Part model, mm, in its own coordinate system. A direction names the side the tool comes from. Give positions to 0.01 mm unless a question says otherwise; leave off trailing zeros. Order: outer loops, then holes, each group sorted by start corner. A loop starts at its lowest first (then second) coordinate and runs counter-clockwise, first axis right, second up. Notation, with made-up numbers: M 22.25,-4.75 L 26.25,-4.75 A33 ccw 26.25,32.25 Z; hole C -9,84.25 d3. An arc over 180 degrees is marked long. Return JSON: item names as keys, results as strings.
from build123d import *

# Parameters (mm, degrees)
SKETCH_1_R      = 2.5
SKETCH_1_R_2    = 1.45
EXTRUDE_2_DEPTH = 3


with BuildPart() as part:
    # 草圖1 → 填料-伸長2 (new body)
    with BuildSketch(Plane.XY):
        with BuildLine():
            ThreePointArc((-56.198698673, 17.411107553), (-54.880679188, 14.229127038), (-51.698698673, 12.911107553))
            Line((-51.698698673, 12.911107553), (-48.698698673, 12.911107553))
            Line((-48.698698673, 12.911107553), (-48.698698673, -10.138892447))
            Line((-48.698698673, -10.138892447), (-51.698698673, -10.138892447))
            ThreePointArc((-51.698698673, -10.138892447), (-54.880679188, -11.456911932), (-56.198698673, -14.638892447))
            Line((-56.198698673, -14.638892447), (-56.198698673, -30.638892447))
            ThreePointArc((-56.198698673, -30.638892447), (-54.83353613, -33.86732769), (-51.566345732, -35.136945659))
            Line((-51.566345732, -35.136945659), (-35.566345732, -35.136945659))
            ThreePointArc((-35.566345732, -35.136945659), (-32.47026343, -33.773729904), (-31.198698673, -30.638892447))
            Line((-31.198698673, -30.638892447), (-31.198698673, -27.638892447))
            Line((-31.198698673, -27.638892447), (23.601301327, -27.638892447))
            Line((23.601301327, -27.638892447), (23.601301327, -30.638892447))
            ThreePointArc((23.601301327, -30.638892447), (24.958086091, -33.914460625), (28.233654268, -35.271245388))
            Line((28.233654268, -35.271245388), (44.233654268, -35.271245388))
            ThreePointArc((44.233654268, -35.271245388), (47.509222446, -33.914460625), (48.866007209, -30.638892447))
            Line((48.866007209, -30.638892447), (48.866007209, -14.638892447))
            ThreePointArc((48.866007209, -14.638892447), (47.547987725, -11.456911932), (44.366007209, -10.138892447))
            Line((44.366007209, -10.138892447), (41.366007209, -10.138892447))
            Line((41.366007209, -10.138892447), (41.366007209, 12.911107553))
            Line((41.366007209, 12.911107553), (44.366007209, 12.911107553))
            ThreePointArc((44.366007209, 12.911107553), (47.547987725, 14.229127038), (48.866007209, 17.411107553))
            Line((48.866007209, 17.411107553), (48.866007209, 33.411107553))
            ThreePointArc((48.866007209, 33.411107553), (47.509222446, 36.686675731), (44.233654268, 38.043460494))
            Line((44.233654268, 38.043460494), (28.233654268, 38.043460494))
            ThreePointArc((28.233654268, 38.043460494), (24.958086091, 36.686675731), (23.601301327, 33.411107553))
            Line((23.601301327, 33.411107553), (23.601301327, 30.411107553))
            Line((23.601301327, 30.411107553), (-30.933992791, 30.411107553))
            Line((-30.933992791, 30.411107553), (-30.933992791, 33.411107553))
            ThreePointArc((-30.933992791, 33.411107553), (-32.290777554, 36.686675731), (-35.566345732, 38.043460494))
            Line((-35.566345732, 38.043460494), (-51.566345732, 38.043460494))
            ThreePointArc((-51.566345732, 38.043460494), (-54.841913909, 36.686675731), (-56.198698673, 33.411107553))
            Line((-56.198698673, 33.411107553), (-56.198698673, 17.411107553))
        make_face()
        with Locations((-51.698698673, -30.638892447)):
            Circle(SKETCH_1_R, mode=Mode.SUBTRACT)
        with Locations((-43.698698673, -30.638892447)):
            Circle(SKETCH_1_R, mode=Mode.SUBTRACT)
        with Locations((-35.698698673, -30.638892447)):
            Circle(SKETCH_1_R, mode=Mode.SUBTRACT)
        with Locations((-51.698698673, -22.638892447)):
            Circle(SKETCH_1_R, mode=Mode.SUBTRACT)
        with Locations((-41.398698673, -22.638892447)):
            Circle(SKETCH_1_R_2, mode=Mode.SUBTRACT)
        with Locations((-51.698698673, -14.638892447)):
            Circle(SKETCH_1_R, mode=Mode.SUBTRACT)
        with Locations((16.601301327, -22.638892447)):
            Circle(SKETCH_1_R_2, mode=Mode.SUBTRACT)
        with Locations((28.233654268, -30.638892447)):
            Circle(SKETCH_1_R, mode=Mode.SUBTRACT)
        with Locations((36.233654268, -30.638892447)):
            Circle(SKETCH_1_R, mode=Mode.SUBTRACT)
        with Locations((44.233654268, -30.638892447)):
            Circle(SKETCH_1_R, mode=Mode.SUBTRACT)
        with Locations((44.233654268, -22.638892447)):
            Circle(SKETCH_1_R, mode=Mode.SUBTRACT)
        with Locations((44.233654268, -14.638892447)):
            Circle(SKETCH_1_R, mode=Mode.SUBTRACT)
        with Locations((-51.566345732, 17.411107553)):
            Circle(SKETCH_1_R, mode=Mode.SUBTRACT)
        with Locations((-51.566345732, 25.411107553)):
            Circle(SKETCH_1_R, mode=Mode.SUBTRACT)
        with Locations((-41.398698673, 26.361107553)):
            Circle(SKETCH_1_R_2, mode=Mode.SUBTRACT)
        with Locations((-51.566345732, 33.411107553)):
            Circle(SKETCH_1_R, mode=Mode.SUBTRACT)
        with Locations((-43.566345732, 33.411107553)):
            Circle(SKETCH_1_R, mode=Mode.SUBTRACT)
        with Locations((-35.566345732, 33.411107553)):
            Circle(SKETCH_1_R, mode=Mode.SUBTRACT)
        with Locations((44.233654268, 17.411107553)):
            Circle(SKETCH_1_R, mode=Mode.SUBTRACT)
        with Locations((16.601301327, 26.361107553)):
            Circle(SKETCH_1_R_2, mode=Mode.SUBTRACT)
        with Locations((44.233654268, 25.411107553)):
            Circle(SKETCH_1_R, mode=Mode.SUBTRACT)
        with Locations((28.233654268, 33.411107553)):
            Circle(SKETCH_1_R, mode=Mode.SUBTRACT)
        with Locations((36.233654268, 33.411107553)):
            Circle(SKETCH_1_R, mode=Mode.SUBTRACT)
        with Locations((44.233654268, 33.411107553)):
            Circle(SKETCH_1_R, mode=Mode.SUBTRACT)
    extrude(amount=EXTRUDE_2_DEPTH)


solid = part.part
Q1. Band-saw the part on B-B (x = 8). Give the cut face in (y, z).
Established:
{"outline": "M -27.64,0 L 30.41,0 L 30.41,3 L -27.64,3 Z"}
Q2. Band-saw the part on C-C (z = 0.5). Give the number of separate pieces and of enclosed holes in the cut face, then the cut area to 3 significant figures.
Established:
{"separate pieces": "1", "enclosed holes": "24", "area": "6,050 mm²"}
Q3. Two-plate mould, pull along Y, no slides. Class faces 4 (the flat face through (-43, 38.043, 1)), 5 (the flat face through (-56.199, -23, 1)), 6 (the cylindrical face through (46.62, -13.89, 1.48)): +Y half, -Y half, draft (parallel to the pull), parting line (faces both ways), or undercut.
Established:
{"face 4": "+Y half", "face 5": "draft", "face 6": "undercut"}
Q4. 3-axis set-ups, long thin cutter, end or side, ignore diameter. For faces 1 (the flat face through (-50, -10.139, 1)), 2 (the cylindrical face through (47.51, 14.19, 1.48)), 3 (the flat face through (36, 38.043, 1)): which of +Z, -Z, +X, -X, +Y, -Y reach the whole face in a straight line?
Established:
{"face 1": "+Z, -Z, -X", "face 2": "+Z, -Z, +X", "face 3": "+Z, -Z, +X, -X, +Y"}
Q5. Band-saw the part on A-A (y = -4). Give the cut face in (x, z), then the cut area to 3 significant figures.
Established:
{"outline": "M -48.7,0 L 41.37,0 L 41.37,3 L -48.7,3 Z", "area": "270 mm²"}
Q6. Probe line 1 along X through (y, z) = (18.5, 1.3); line 2 along Y through (x, z) = (-41.5, 2.05); line 3 along Y through (x, z) = (-34, 1.4). List the from-to ranges inside material, lowest first.
Established:
{"line 1": "x = -56.2 to -53.82, -49.32 to 41.98, 46.48 to 48.87", "line 2": "y = -35.14 to -31.83, -29.45 to -24.09, -21.19 to 24.91, 27.81 to 32, 34.82 to 38.04", "line 3": "y = -34.81 to -32.47, -28.8 to 31.46, 35.36 to 37.77"}
Q7. Pin check, flat tips, straight feed: pin 1 (4 mm diameter, centred on x = 16.6, y = -22.64, fed in from +Z); pin 2 (1.5 mm diameter, centred on x = -35.5, z = 1.5, fed in from -Y). Stop position of each tip, or through.
Established:
{"pin 1": "stops at z = 3", "pin 2": "stops at y = -35.14"}
